```python
from build123d import *

# Parameters (mm, degrees)
F0_W     = 20
F0_H     = 110
F1_DEPTH = 15
F2_R     = 3
F3_DEPTH = 10
F4_R     = 4
F5_R     = 2


with BuildPart() as f1:
    # F0 (on Top) → F1 (new body)
    with BuildSketch(Plane.XY):
        with Locations((0, 35)):
            Rectangle(F0_W, F0_H)
    extrude(amount=F1_DEPTH)

    # F2 (on Top) → F3 (cut)
    with BuildSketch(Plane.XY):
        Circle(F2_R)
    extrude(amount=F3_DEPTH, mode=Mode.SUBTRACT)

    # F4
    f4_edges = [f1.edges().sort_by_distance(p)[0] for p in [
        (10, 35, 15),
        (-10, 35, 15),
        (10, 35, 0),
        (-10, 35, 0),
    ]]
    fillet(f4_edges, radius=F4_R)

    # F5
    f5_edges = [f1.edges().sort_by_distance(p)[0] for p in [
        (8.828427, 90, 1.171573),
    ]]
    fillet(f5_edges, radius=F5_R)


solid = f1.part
```
Input: part model. Units: mm. Frame: model coordinates. Give positions to 0.01 mm unless a question says otherwise; leave off trailing zeros. Order: outer loops, then holes, each group sorted by start corner. A loop starts at its lowest first (then second) coordinate and runs counter-clockwise, first axis right, second up.
1. Line query: probe 1 along Y at (x, z) = (0, 5.25); probe 2 along X at (y, z) = (62.5, 3.75); probe 3 along X at (y, z) = (63.5, 3.25). Output: solid intervals per line, ascending.
Computed:
probe 1: y = -20 to -3, 3 to 90
probe 2: x = -9.99 to 9.99
probe 3: x = -9.93 to 9.93
2. Cut plane A-A (y = 75.5). Return loops of the section in (x, z), and give its area (3 significant figures).
Computed:
outline: (-10, 4) arc R4 ccw to (-6, 0) - (6, 0) arc R4 ccw to (10, 4) - (10, 11) arc R4 ccw to (6, 15) - (-6, 15) arc R4 ccw to (-10, 11) - close
area: 286 mm2
3. Cut plane C-C (y = 0). Return loops of the section in (x, z).
Computed:
outline: (-10, 4) arc R4 ccw to (-6, 0) - (-3, 0) - (-3, 10) - (3, 10) - (3, 0) - (6, 0) arc R4 ccw to (10, 4) - (10, 11) arc R4 ccw to (6, 15) - (-6, 15) arc R4 ccw to (-10, 11) - close
4. Pin query (flat end, axial travel): pin 1 Ø1.8 at (x, y) = (1.5, 0) entering from -Z. Return the tip coordinate at first contact, or that it passes through.
Computed:
pin 1: stops at z = 10
5. Cut plane B-B (x = 0). Return loops of the section in (y, z), and give its area (3 significant figures).
Computed:
outline: (-20, 0) - (-3, 0) - (-3, 10) - (3, 10) - (3, 0) - (88, 0) arc R2 ccw to (90, 2) - (90, 13) arc R2 ccw to (88, 15) - (-20, 15) - close
area: 1,590 mm2
6. Draft query along Y for faces 1 (the face through (0, 0, 10)), 2 (the face through (8.797, 34.756, 13.859)), 3 (the face through (9.4, 89.43, 7.55)), 4 (the face through (-3, 0, 5)). Return one class per face: released by +Y, released by -Y, zero draft, split by the parting line, or undercut.
Computed:
face 1: undercut
face 2: zero draft
face 3: released by +Y
face 4: undercut
